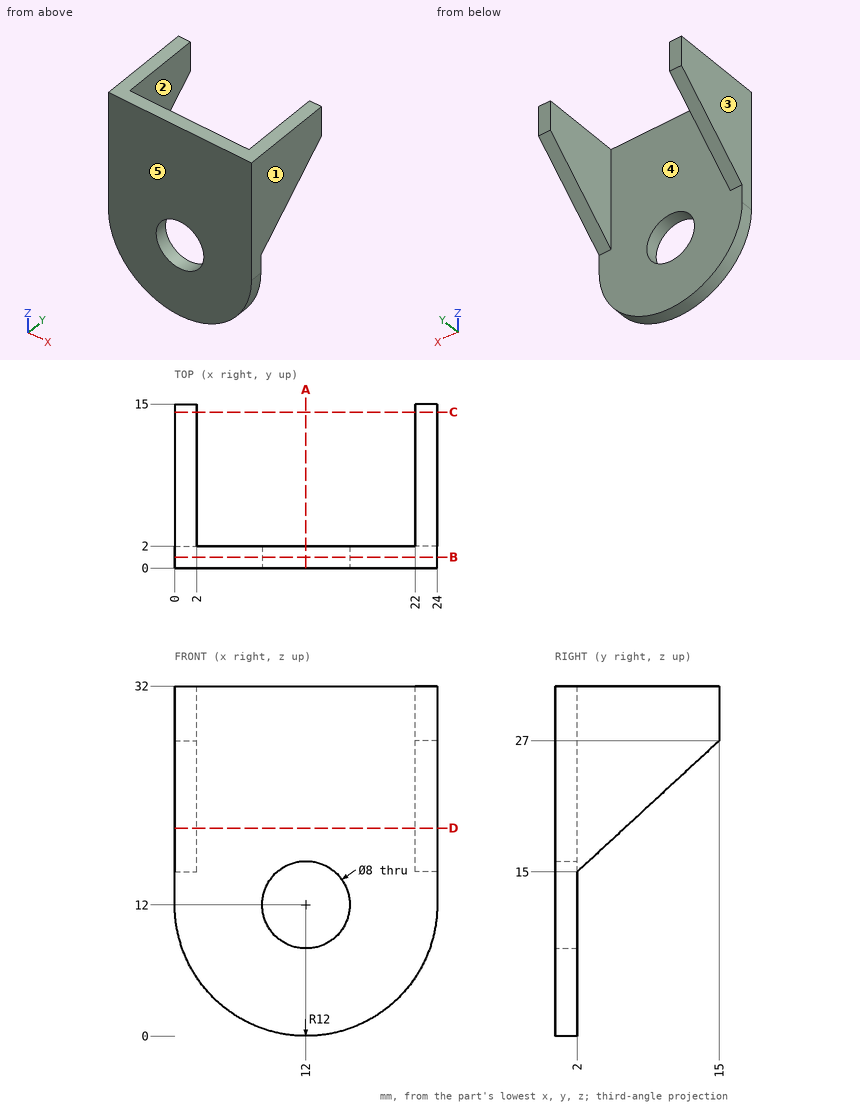
Print and shaded views of the part. All mm, measured from the part's lowest x, y and z. A direction names the side the tool comes from. Coordinates: 2 decimals unless noted, no trailing zeros. Order: outer loops, then holes, each group sorted by start corner. A loop starts at its lowest first (then second) coordinate and runs counter-clockwise, first axis right, second up. Notation, with made-up numbers: (62.5, 20) -> (104.5, 20) arc R20 ccw to (104.5, 37) -> close; hole circle Ø11 at (88, 34). An arc over 180 degrees is marked (long way). Use one line per item in the form item = value. Start each with the question number.
1) Band-saw the part on D-D on z = 19. Give the cut face in (x, y), then the cut area to 3 significant figures.
2) Band-saw the part on A-A on x = 12. Give the cut face in (y, z), then the cut area to 3 significant figures.
3) Band-saw the part on C-C on y = 14.25. Give the cut face in (x, z).
4) Drop flat-ended pins along their axis: pin 1 (5 mm diameter, centred on x = 19, y = 10.5, fed in from +Z); pin 2 (1 mm diameter, centred on x = 12, z = 24.5, fed in from +Y). Give the stop position or say it passes through.
5) Band-saw the part on B-B on y = 1. Give the cut face in (x, z).
6) Tool access for the marked faces 1 and 2: list every direction of +Z, -Z, +X, -X, +Y, -Y with a clear straight run to the whole face (end or side of a thin tool).
7) Pull direction Y, two halves, no side cores. Call the marked faces 3, 4 and 5: +Y half, -Y half, draft (parallel to the pull), parting line (faces both ways), or undercut.
8) Drill centre lines: L1, parallel to X at y = 12, z = 26; L2, parallel to X at y = 1.2, z = 12; L3, parallel to Y at x = 16, z = 27.5. Where is each one in solid material? Low to high. Write a range as [from, to].
Entries:
q1.outline = (0, 0) -> (24, 0) -> (24, 6.33) -> (22, 6.33) -> (22, 2) -> (2, 2) -> (2, 6.33) -> (0, 6.33) -> close
q1.area = 65.3 mm2
q2.outline = (0, 0) -> (2, 0) -> (2, 8) -> (0, 8) -> close; (0, 16) -> (2, 16) -> (2, 32) -> (0, 32) -> close
q2.area = 48.0 mm2
q3.outline = (0, 26.31) -> (2, 26.31) -> (2, 32) -> (0, 32) -> close; (22, 26.31) -> (24, 26.31) -> (24, 32) -> (22, 32) -> close
q4.pin_1 = through
q4.pin_2 = 2
q5.outline = (0, 12) arc R12 ccw to (24, 12) -> (24, 32) -> (0, 32) -> close; hole circle Ø8 at (12, 12)
q6.face_1 = +Z, -Z, +X, +Y, -Y
q6.face_2 = +Z, -Z, +Y
q7.face_3 = draft
q7.face_4 = +Y half
q7.face_5 = -Y half
q8.L1 = [0, 2], [22, 24]
q8.L2 = [0, 8], [16, 24]
q8.L3 = [0, 2]
